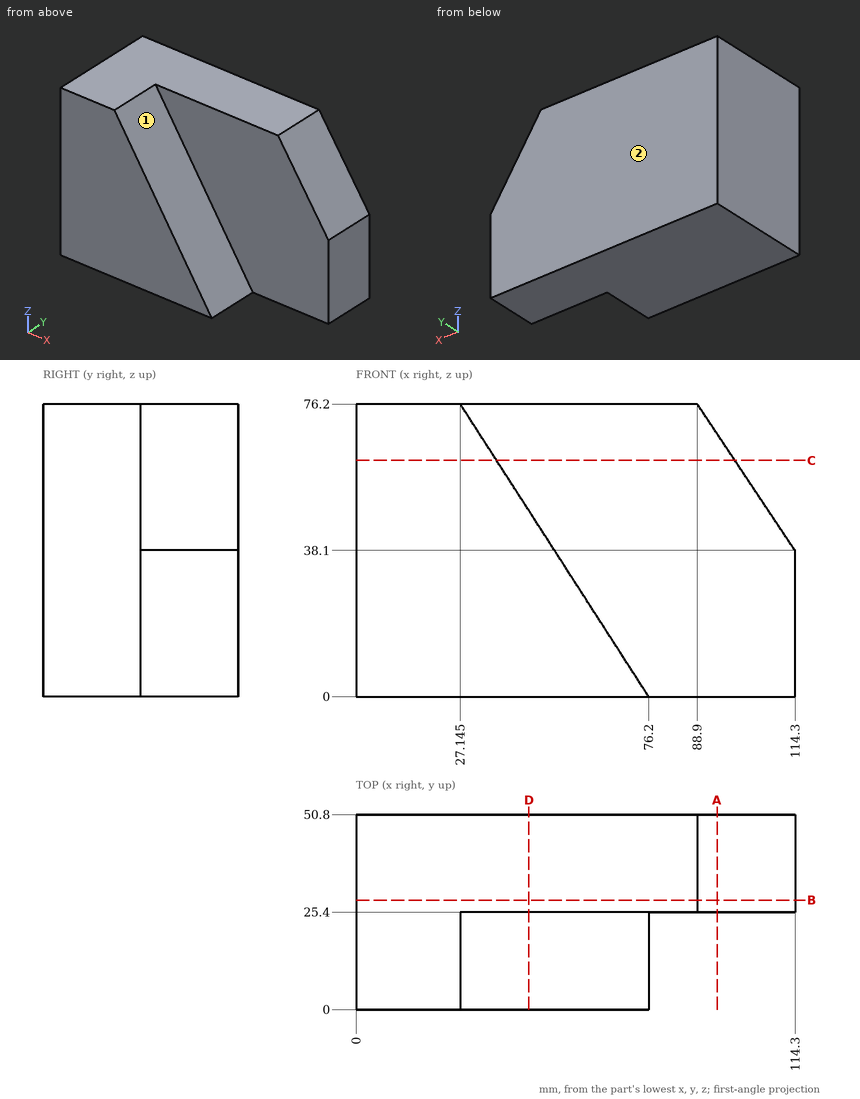
Source: three-view drawing plus pictorial views. Frame: mm from the lowest corner of the part. A direction names the side the tool comes from. Coordinates: 2 decimals unless noted, no trailing zeros. Order: outer loops, then holes, each group sorted by start corner. A loop starts at its lowest first (then second) coordinate and runs counter-clockwise, first axis right, second up. Notation, with made-up numbers: M -22.75,19 L -5.75,19 A20 cw -5.75,45 Z; hole C 56,-5.5 d4. An arc over 180 degrees is marked long. Write each question's results on one line, items separated by ' | '. Start each with the question number.
1. Pin query (flat end, axial travel): pin 1 (12 mm diameter, centred on x = 88.5, z = 29, fed in from -Y). Return the tip coordinate at first contact, or that it passes through.
2. Section D-D, the plane x = 45. Return the cut outline in (y, z) (3 decimals), then the cut area to 3 significant figures.
3. Section B-B, the plane y = 28.5. Return the cut outline in (x, z).
4. Reachability of the marked faces 1 and 2 from +Z, -Z, +X, -X, +Y, -Y: full face, straight path, thin tool, end or side. Return the list, or none.
5. Material intervals for L1, parallel to Y at x = 48, z = 51; L2, parallel to X at y = 14, z = 39.5; L3, parallel to Z at x = 63, y = 15.5 (1 decimal), sorted ascending.
6. Section C-C, the plane z = 61.5. Return the cut outline in (x, y).
7. Section A-A, the plane x = 94. Return the cut outline in (y, z), then the cut area to 3 significant figures.
Solution:
1) pin 1: y = 25.4
2) outline: M 0,0 L 50.8,0 L 50.8,76.2 L 25.4,76.2 L 25.4,48.465 L 0,48.465 Z | area: 3,170 mm²
3) outline: M 0,0 L 114.3,0 L 114.3,38.1 L 88.9,76.2 L 0,76.2 Z
4) face 1: +Z, +X, -Y | face 2: +Z, -Z, +X, -X, +Y
5) L1: 25.4 to 50.8 | L2: 0 to 50.77 | L3: 0 to 20.5
6) outline: M 0,0 L 36.61,0 L 36.61,25.4 L 98.7,25.4 L 98.7,50.8 L 0,50.8 Z
7) outline: M 25.4,0 L 50.8,0 L 50.8,68.55 L 25.4,68.55 Z | area: 1,740 mm²
